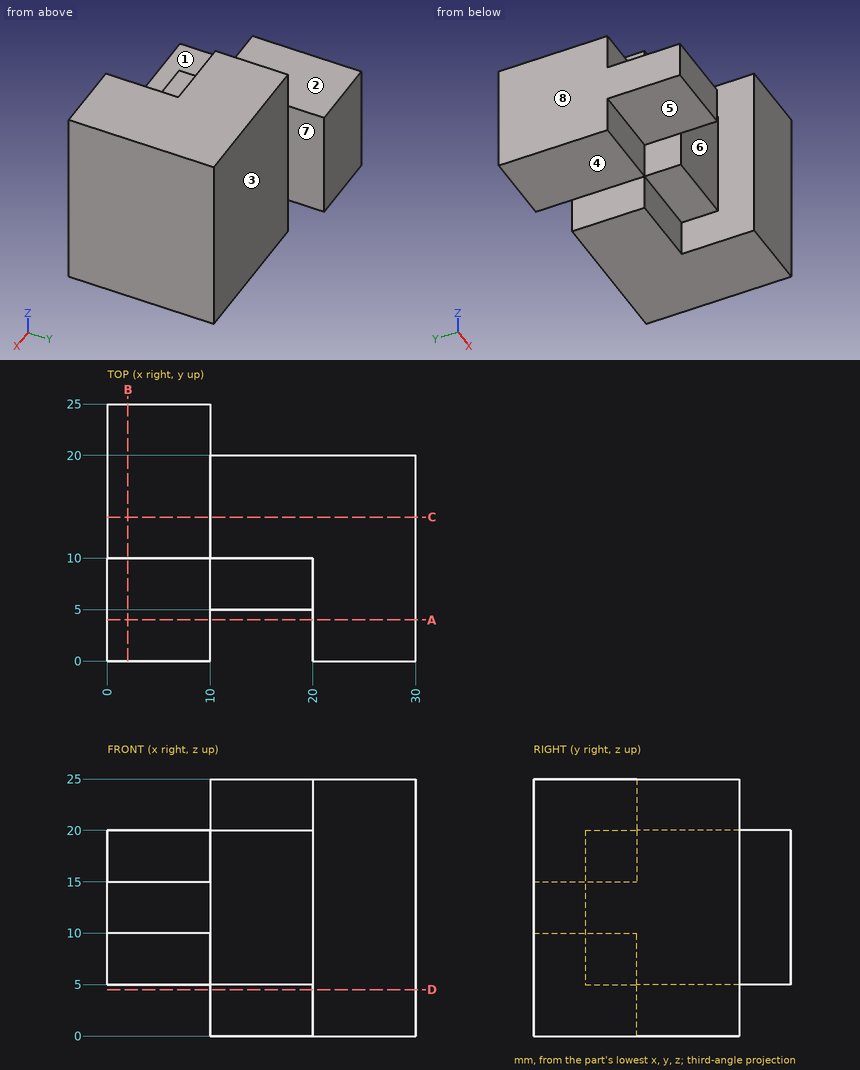
Geometry check sheet. Reference: drawing and pictorial views, mm from the part's lowest x, y, z. A direction names the side the tool comes from. Coordinates: 2 decimals unless noted, no trailing zeros. Order: outer loops, then holes, each group sorted by start corner. A loop starts at its lowest first (then second) coordinate and runs counter-clockwise, first axis right, second up. Notation, with made-up numbers: (76.5, -20.75) - (86.5, -20.75) arc R19 ccw to (86.5, -1.75) - close; hole circle Ø3 at (16.25, -35.75). An arc over 180 degrees is marked (long way). One line per item, written item: value.
(1) Sectioned sample at B-B (x = 2). Enter the section's corners in (y, z), and give its area (3 significant figures).
Data:
outline: (0, 10) - (10, 10) - (10, 5) - (25, 5) - (25, 20) - (10, 20) - (10, 15) - (0, 15) - close
area: 275 mm^2
(2) Sectioned sample at D-D (z = 4.5). Enter the section's corners in (x, y), and give its area (3 significant figures).
Data:
outline: (10, 10) - (20, 10) - (20, 0) - (30, 0) - (30, 20) - (10, 20) - close
area: 300 mm^2
(3) Access from +Z, -Z, +X, -X, +Y, -Y to the whole of each face (thin tool, end or side, straight path). Record for the marked faces 1, 2, 3, 4 and 5.
Data:
face 1: +Z, -X, -Y
face 2: +Z, -X, +Y, -Y
face 3: +Z, -Z, +X, +Y
face 4: -Z, -X, +Y, -Y
face 5: -Z, -X, -Y
(4) Depth check by flat-ended pin: pin 1 Ø1.5 at (x, z) = (10, 3) entering from -Y; pin 2 Ø10 at (x, z) = (25.5, 8) entering from +Y; pin 3 Ø5.5 at (y, z) = (7, 6.5) entering from -X. Enter the tip coordinate at first touch or a pass-through.
Data:
pin 1: stops at y = 10
pin 2: stops at y = 20
pin 3: stops at x = 10
(5) Sectioned sample at A-A (y = 4). Enter the section's corners in (x, z), and give its area (3 significant figures).
Data:
outline: (0, 10) - (10, 10) - (10, 15) - (0, 15) - close; (20, 0) - (30, 0) - (30, 25) - (20, 25) - close
area: 300 mm^2
(6) Thickness scan on probe 1 along X at (y, z) = (10.75, 23.5); probe 2 along Y at (x, z) = (28, 8.25); probe 3 along Z at (x, y) = (11, 8.5). Record the ranges inside material, lowest first. Write a range as from..to.
Data:
probe 1: x = 10..30
probe 2: y = 0..20
probe 3: z = 5..20
(7) Release check for a two-part mould opening along X. For the marked faces 6, 7 and 8 record: +X half, -X half, draft (parallel to the pull), parting line (faces both ways), or undercut.
Data:
face 6: undercut
face 7: +X half
face 8: -X half
(8) Sectioned sample at C-C (y = 14). Enter the section's corners in (x, z).
Data:
outline: (0, 5) - (10, 5) - (10, 0) - (30, 0) - (30, 25) - (10, 25) - (10, 20) - (0, 20) - close
